Check sheet for the modelled part. Datum: model origin and axes. Units: mm. Face numbers are marked on the shaded views. Give positions to 0.01 mm unless a question says otherwise; leave off trailing zeros. Order: outer loops, then holes, each group sorted by start corner. A loop starts at its lowest first (then second) coordinate and runs counter-clockwise, first axis right, second up.
Item 1: Sectioned sample at C-C on y = -2.75. Record the boundary of the cut face in (x, z), and give its area (3 significant figures).
Item 2: Sectioned sample at B-B on z = 47. Record the boundary of the cut face in (x, y), and give its area (3 significant figures).
Item 3: Gauge pin test, flat ends, axial feed: P1, Ø5, axis at x = -5, y = 6, coming from the +Z side; P2, Ø6, axis at y = 1.5, z = -33.5, coming from the -X side; P3, Ø8, axis at y = 0, z = -29.5, coming from the -X side. Record the tip position at first contact, or that the pin passes through.
Item 4: Sectioned sample at A-A on x = 0. Record the boundary of the cut face in (y, z), and give its area (3 significant figures).
Item 5: Sectioned sample at D-D on z = 0. Record the boundary of the cut face in (x, y), and give its area (3 significant figures).
Item 6: Material ranges on line 1 along Z through (x, y) = (1.5, 6); line 2 along X through (y, z) = (5.5, 42); line 3 along Y through (x, z) = (-9, -52.5), recorded low to high.
Item 7: Release check for a two-part mould opening along Z. For the marked faces 1, 2, 3 and 4 record: released by +Z, released by -Z, zero draft, split by the parting line, or undercut.
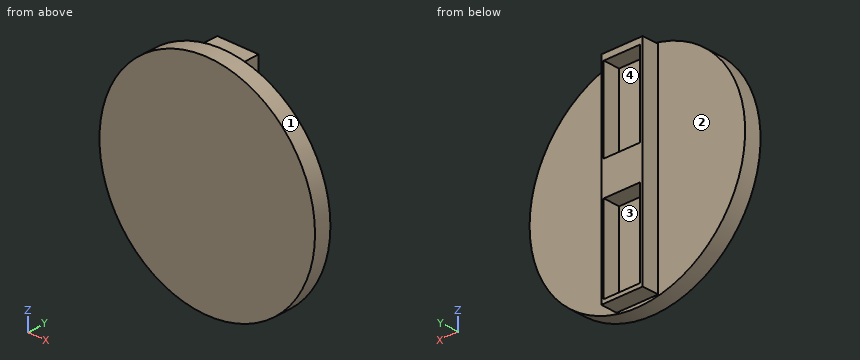
from build123d import *

# Parameters (mm, degrees)
SKETCH1_W           = 25
SKETCH1_H           = 126
SKETCH1_W_2         = 22
SKETCH1_H_2         = 50.698113208
SKETCH1_H_3         = 49.301886792
BOSS_EXTRUDE1_DEPTH = 10
SKETCH2_R           = 65
BOSS_EXTRUDE2_DEPTH = 10


with BuildPart() as part:
    # Sketch1 → Boss-Extrude1 (new body)
    with BuildSketch(Plane(origin=(0, 0, 0), x_dir=(1, 0, 0), z_dir=(0, 1, 0))):
        Rectangle(SKETCH1_W, SKETCH1_H)
        with Locations((0, 35.349056604)):
            Rectangle(SKETCH1_W_2, SKETCH1_H_2, mode=Mode.SUBTRACT)
        with Locations((0, -34.650943396)):
            Rectangle(SKETCH1_W_2, SKETCH1_H_3, mode=Mode.SUBTRACT)
    extrude(amount=BOSS_EXTRUDE1_DEPTH)

    # Sketch2 → Boss-Extrude2 (add)
    with BuildSketch(Plane(origin=(0, 0, 0), x_dir=(1, 0, 0), z_dir=(0, 1, 0))):
        Circle(SKETCH2_R)
    extrude(amount=-BOSS_EXTRUDE2_DEPTH)


solid = part.part
Report:
1. outline: circle Ø130 at (0, 0)
1. area: 13,300 mm2
2. outline: (-44.9, -10) - (44.9, -10) - (44.9, 0) - (12.5, 0) - (12.5, 10) - (11, 10) - (11, 0) - (-11, 0) - (-11, 10) - (-12.5, 10) - (-12.5, 0) - (-44.9, 0) - close
2. area: 928 mm2
3. P1: stops at z = 63
3. P2: stops at x = -57.18
3. P3: stops at x = -59.79
4. outline: (-10, -65) - (0, -65) - (0, -63) - (10, -63) - (10, -60.7) - (0, -60.7) - (0, -10) - (10, -10) - (10, 10) - (0, 10) - (0, 59.3) - (10, 59.3) - (10, 63) - (0, 63) - (0, 65) - (-10, 65) - close
4. area: 1,560 mm2
5. outline: (-65, -10) - (65, -10) - (65, 0) - (12.5, 0) - (12.5, 10) - (-12.5, 10) - (-12.5, 0) - (-65, 0) - close
5. area: 1,550 mm2
6. line 1: z = -63 to -60.7, -10 to 10, 59.3 to 63
6. line 2: x = -12.5 to -11, 11 to 12.5
6. line 3: y = -10 to 0
7. face 1: split by the parting line
7. face 2: zero draft
7. face 3: undercut
7. face 4: undercut
